CAD build for the part. Positions are in the model's coordinates, mm. A direction names the side the tool comes from. Coordinates: 2 decimals unless noted, no trailing zeros. Order: outer loops, then holes, each group sorted by start corner. A loop starts at its lowest first (then second) coordinate and runs counter-clockwise, first axis right, second up. Notation, with made-up numbers: (35.25, 71) -> (70.25, 71) arc R19 cw to (70.25, 103) -> close; hole circle Ø2 at (-29, 4.25). An arc over 180 degrees is marked (long way). Use one line per item in the form item = value. Start each with the question number.
from build123d import *

# Parameters (mm, degrees)
F0_R     = 7.5
F1_DEPTH = 5


with BuildPart() as f1:
    # F0 (on Top) → F1 (new body)
    with BuildSketch(Plane.XY):
        with BuildLine():
            Line((52.206931, 24.999788), (-21.739577, 24.999788))
            ThreePointArc((-21.739577, 24.999788), (-34.239524, 12.463405), (-21.66681, 0))
            ThreePointArc((-21.66681, 0), (-15.027254, 1.954897), (-10.445656, 7.142797))
            ThreePointArc((-10.445656, 7.142797), (-8.600729, 9.225753), (-5.928088, 10))
            Line((-5.928088, 10), (52.206931, 10))
            Line((52.206931, 10), (52.206931, 24.999788))
        make_face()
        with Locations((-21.739577, 12.499788)):
            Circle(F0_R, mode=Mode.SUBTRACT)
    extrude(amount=F1_DEPTH)


solid = f1.part
1) Cut at D-D on x = 14. Give the cut face in (y, z).
2) Two-plate mould, pull along X, no slides. Class faces 3 (the face through (16, 25, 2)), 4 (the face through (-22.716, 19.936, 2.465)), 5 (the face through (-8.634, 9.205, 2.465)): released by +X, released by -X, zero draft, split by the parting line, or undercut.
3) Drop flat-ended pins along their axis: P1, Ø1.5, axis at x = 31, z = 2, coming from the -Y side; P2, Ø1, axis at y = 8.5, z = 2, coming from the +X side; P3, Ø1, axis at y = 15, z = 2.5, coming from the -X side. Give the stop position or say it passes through.
4) 3-axis set-ups, long thin cutter, end or side, ignore diameter. For faces 1 (the face through (23, 10, 2)), 2 (the face through (8, 15, 0)): which of +Z, -Z, +X, -X, +Y, -Y reach the whole face in a straight line?
5) Probe L1, parallel to Y at x = -22, z = 3.7; L2, parallel to Y at x = 31, z = 3.4; L3, parallel to X at y = 8, z = 2.5. List the from-to ranges inside material, lowest first.
6) Cut at A-A on y = 15.25. Give the cut face in (x, z).
7) Cut at C-C on z = 3.7. Give the cut face in (x, y).
8) Cut at B-B on x = -23. Give the cut face in (y, z), then the cut area to 3 significant figures.
Values follow:
q1.outline = (10, 0) -> (25, 0) -> (25, 5) -> (10, 5) -> close
q2.face_3 = zero draft
q2.face_4 = undercut
q2.face_5 = released by +X
q3.P1 = 10
q3.P2 = -8.93
q3.P3 = -34.08
q4.face_1 = +Z, -Z, +X, -Y
q4.face_2 = -Z, +X, -X, +Y, -Y
q5.L1 = 0 to 5, 20 to 25
q5.L2 = 10 to 25
q5.L3 = -33.4 to -27.74, -15.74 to -9.93
q6.outline = (-33.93, 0) -> (-28.72, 0) -> (-28.72, 5) -> (-33.93, 5) -> close; (-14.76, 0) -> (52.21, 0) -> (52.21, 5) -> (-14.76, 5) -> close
q7.outline = (-21.74, 25) arc R12.5 ccw (long way) to (-21.67, 0) arc R12.5 ccw to (-10.45, 7.14) arc R5 cw to (-5.93, 10) -> (52.21, 10) -> (52.21, 25) -> close; hole circle Ø15 at (-21.74, 12.5)
q8.outline = (0.06, 0) -> (5.11, 0) -> (5.11, 5) -> (0.06, 5) -> close; (19.89, 0) -> (24.94, 0) -> (24.94, 5) -> (19.89, 5) -> close
q8.area = 50.4 mm^2
